```python
from build123d import *

# Parameters (mm, degrees)
SKETCH1_W           = 151
SKETCH1_H           = 100
BOSS_EXTRUDE1_DEPTH = 3
SKETCH3_W           = 1.5
SKETCH3_H           = 3.5
CUT_EXTRUDE1_DEPTH  = 182.13530854
SKETCH4_W           = 10
SKETCH4_H           = 100
BOSS_EXTRUDE2_DEPTH = 3
SKETCH5_R           = 3
SKETCH5_R_2         = 1.75
CUT_EXTRUDE2_DEPTH  = 190.552103655
FILLET1_R           = 3
FILLET2_R           = 3
SKETCH6_W           = 3
SKETCH6_H           = 5
SKETCH6_H_2         = 10
SKETCH6_W_2         = 10
SKETCH6_H_3         = 3
CUT_EXTRUDE3_DEPTH  = 190.552103655


with BuildPart() as part:
    # Sketch1 → Boss-Extrude1 (new body)
    with BuildSketch(Plane(origin=(0, 0, 0), x_dir=(1, 0, 0), z_dir=(0, 1, 0))):
        with Locations((75.5, -50)):
            Rectangle(SKETCH1_W, SKETCH1_H)
    extrude(amount=BOSS_EXTRUDE1_DEPTH)

    # Sketch3 → Cut-Extrude1 (cut, through all)
    with BuildSketch(Plane.XZ):
        with Locations((40.75, 86)):
            Rectangle(SKETCH3_W, SKETCH3_H)
        with Locations((48.25, 86)):
            Rectangle(SKETCH3_W, SKETCH3_H)
        with Locations((129.25, 86)):
            Rectangle(SKETCH3_W, SKETCH3_H)
        with Locations((136.75, 86)):
            Rectangle(SKETCH3_W, SKETCH3_H)
    extrude(amount=-CUT_EXTRUDE1_DEPTH, mode=Mode.SUBTRACT)

    # Sketch4 → Boss-Extrude2 (add, through all)
    with BuildSketch(Plane.XZ):
        with Locations((156, 50)):
            Rectangle(SKETCH4_W, SKETCH4_H)
    extrude(amount=-BOSS_EXTRUDE2_DEPTH)

    # Sketch5 → Cut-Extrude2 (cut, through all)
    with BuildSketch(Plane.XZ):
        with Locations(Location((155, 50, 0), (0, 0, 270))):
            Circle(SKETCH5_R)
        with Locations(Location((155, 90, 0), (0, 0, 270))):
            Circle(SKETCH5_R_2)
        with Locations(Location((155, 10, 0), (0, 0, 270))):
            Circle(SKETCH5_R_2)
    extrude(amount=-CUT_EXTRUDE2_DEPTH, mode=Mode.SUBTRACT)

    # Fillet1
    fillet1_edges = [part.edges().sort_by_distance(p)[0] for p in [
        (0, 1.5, 0),
        (0, 1.5, 100),
    ]]
    fillet(fillet1_edges, radius=FILLET1_R)

    # Fillet2
    fillet2_edges = [part.edges().sort_by_distance(p)[0] for p in [
        (161, 1.5, 100),
        (161, 1.5, 0),
    ]]
    fillet(fillet2_edges, radius=FILLET2_R)

    # Sketch6 → Cut-Extrude3 (cut, through all)
    with BuildSketch(Plane(origin=(0, 3, 0), x_dir=(1, 0, 0), z_dir=(0, 1, 0))):
        with Locations((146.5, -91.5)):
            Rectangle(SKETCH6_W, SKETCH6_H)
        with Locations((146.5, -78.5)):
            Rectangle(SKETCH6_W, SKETCH6_H)
        with Locations((146.5, -51)):
            Rectangle(SKETCH6_W, SKETCH6_H_2)
        with Locations((146.5, -31)):
            Rectangle(SKETCH6_W, SKETCH6_H_2)
        with Locations((146.5, -11)):
            Rectangle(SKETCH6_W, SKETCH6_H_2)
        with Locations((135.5, -4.5)):
            Rectangle(SKETCH6_W_2, SKETCH6_H_3)
        with Locations((115.5, -4.5)):
            Rectangle(SKETCH6_W_2, SKETCH6_H_3)
        with Locations((95.5, -4.5)):
            Rectangle(SKETCH6_W_2, SKETCH6_H_3)
        with Locations((75.5, -4.5)):
            Rectangle(SKETCH6_W_2, SKETCH6_H_3)
        with Locations((55.5, -4.5)):
            Rectangle(SKETCH6_W_2, SKETCH6_H_3)
        with Locations((35.5, -4.5)):
            Rectangle(SKETCH6_W_2, SKETCH6_H_3)
        with Locations((15.5, -4.5)):
            Rectangle(SKETCH6_W_2, SKETCH6_H_3)
        with Locations((4.5, -11)):
            Rectangle(SKETCH6_W, SKETCH6_H_2)
        with Locations((4.5, -31)):
            Rectangle(SKETCH6_W, SKETCH6_H_2)
        with Locations((4.5, -51)):
            Rectangle(SKETCH6_W, SKETCH6_H_2)
        with Locations((4.5, -78.5)):
            Rectangle(SKETCH6_W, SKETCH6_H)
        with Locations((4.5, -91.5)):
            Rectangle(SKETCH6_W, SKETCH6_H)
        with Locations((15.5, -95.5)):
            Rectangle(SKETCH6_W_2, SKETCH6_H_3)
        with Locations((35.5, -95.5)):
            Rectangle(SKETCH6_W_2, SKETCH6_H_3)
        with Locations((55.5, -95.5)):
            Rectangle(SKETCH6_W_2, SKETCH6_H_3)
        with Locations((75.5, -95.5)):
            Rectangle(SKETCH6_W_2, SKETCH6_H_3)
        with Locations((95.5, -95.5)):
            Rectangle(SKETCH6_W_2, SKETCH6_H_3)
        with Locations((115.5, -95.5)):
            Rectangle(SKETCH6_W_2, SKETCH6_H_3)
        with Locations((135.5, -95.5)):
            Rectangle(SKETCH6_W_2, SKETCH6_H_3)
    extrude(amount=-CUT_EXTRUDE3_DEPTH, mode=Mode.SUBTRACT)


solid = part.part
```
Geometry check sheet. Reference: the model listing, model coordinates, mm. A direction names the side the tool comes from. Coordinates: 2 decimals unless noted, no trailing zeros. Order: outer loops, then holes, each group sorted by start corner. A loop starts at its lowest first (then second) coordinate and runs counter-clockwise, first axis right, second up.
Item 1: Section check D-D (y = 2.4). Count the separate pieces of the cut face and the enclosed holes in it, plus the area to 3 significant figures.
Item 2: Section check A-A (z = 50). Enter the section's corners in (x, y).
Item 3: Scan lines: line 1 along X through (y, z) = (0.8, 90); line 2 along Z through (x, y) = (17, 2.55); line 3 along Z through (x, y) = (155, 2.1). Record each from-to range of solid material in increasing order.
Item 4: Section check C-C (z = 78.5). Enter the section's corners in (x, y), plus the area to 3 significant figures.
Item 5: Section check B-B (x = 155). Enter the section's corners in (y, z), plus the area to 3 significant figures.
Item 6: Mould release check, pull along X, two halves, no side actions. Record for faces 1 (the cylindrical face through (0.9, 1.52, 0.86)), 2 (the flat face through (146, 2, 94)), 3 (the flat face through (47.5, 1, 86)): released by +X, released by -X, zero draft, split by the parting line, or undercut.
Item 7: Tool access check on faces 4 (the flat face through (0, 1, 51)), 5 (the flat face through (10.5, 2, 96)). Record the directions out of +Z, -Z, +X, -X, +Y, -Y that give a thin tool (end or side, any length) a straight path to the whole face; none if there is none.
Check sheet entries:
1. separate pieces: 1
1. enclosed holes: 31
1. area: 15,400 mm2
2. outline: (0, 0) - (3, 0) - (3, 3) - (0, 3) - close; (6, 0) - (145, 0) - (145, 3) - (6, 3) - close; (148, 0) - (152, 0) - (152, 3) - (148, 3) - close; (158, 0) - (161, 0) - (161, 3) - (158, 3) - close
3. line 1: x = 0 to 3, 6 to 145, 148 to 153.25, 156.75 to 161
3. line 2: z = 0 to 3, 6 to 94, 97 to 100
3. line 3: z = 0 to 8.25, 11.75 to 47, 53 to 88.25, 91.75 to 100
4. outline: (0, 0) - (3, 0) - (3, 3) - (0, 3) - close; (6, 0) - (145, 0) - (145, 3) - (6, 3) - close; (148, 0) - (161, 0) - (161, 3) - (148, 3) - close
4. area: 465 mm2
5. outline: (0, 0) - (3, 0) - (3, 8.25) - (0, 8.25) - close; (0, 11.75) - (3, 11.75) - (3, 47) - (0, 47) - close; (0, 53) - (3, 53) - (3, 88.25) - (0, 88.25) - close; (0, 91.75) - (3, 91.75) - (3, 100) - (0, 100) - close
5. area: 261 mm2
6. face 1: released by -X
6. face 2: undercut
6. face 3: undercut
7. face 4: +Z, -Z, -X, +Y, -Y
7. face 5: +Y, -Y
